Geometry check sheet. Reference: the model listing, model coordinates, mm. Round coordinates to 2 decimals unless told otherwise and drop trailing zeros. Loops run counter-clockwise (first coordinate to the right, second up) from the corner with the lowest first, then second, coordinate; pieces in that order, holes last. Notation, with made-up numbers: (-21, 20.5) -> (24, 20.5) arc R22 ccw to (24, 28.5) -> close; hole circle Ø7 at (17.5, -11). An arc over 180 degrees is marked (long way). Use a Markdown table: item, result. Add a question column.
Q1. Sectioned sample at D-D, the plane x = 1518.5. Enter the section's corners in (y, z).
Q2. Release check for a two-part mould opening along Z. For faces 1 (the face through (1175, -9, 335)), 2 (the face through (1360, -9, 10)), 3 (the face through (1361, -9, 344)), 4 (the face through (1360, -9, 670)) record: released by +Z, released by -Z, zero draft, split by the parting line, or undercut.
Q3. Material ranges on L1, parallel to X at y = -10, z = 461.5; L2, parallel to Y at x = 1386, z = 499.5; L3, parallel to Z at x = 1360, y = -13, recorded low to high.
Q4. Sectioned sample at A-A, the plane z = 313. Enter the section's corners in (x, y), then the cut area to 4 significant figures.
Q5. Sectioned sample at C-C, the plane z = 604.5. Enter the section's corners in (x, y), then the cut area to 4 significant figures.
Q6. Sectioned sample at B-B, the plane x = 1356. Enter the section's corners in (y, z), then the cut area to 3 significant figures.
```python
from build123d import *

# Parameters (mm, degrees)
CLONE2D002_W    = 375
CLONE2D002_H    = 660
PAD011_DEPTH    = 19
SKETCH027_W     = 225
SKETCH027_H     = 510
POCKET011_DEPTH = 10


with BuildPart() as part:
    # Clone2D002 → Pad011 (new body)
    with BuildSketch(Plane.XZ):
        with Locations((187.5, 330)):
            Rectangle(CLONE2D002_W, CLONE2D002_H)
    extrude(amount=PAD011_DEPTH)

    # Sketch027 (on Face6 of Pad011) → Pocket011 (cut)
    with BuildSketch(Plane.XZ.offset(19)):
        with Locations((187.5, 330)):
            Rectangle(SKETCH027_W, SKETCH027_H)
    extrude(amount=-POCKET011_DEPTH, mode=Mode.SUBTRACT)

    # Clone2D003 (on Face1 of Pocket011) → Revolution001 (revolve)
    with BuildSketch(Plane(origin=(40, -19, 330), x_dir=(-1, 0, 0), z_dir=(0, 0, -1))):
        with BuildLine():
            Line((0, 0), (0, -20))
            add(Edge.make_bspline(
                [(0, -20), (-18, -20), (-18, -9.133286), (-4.506424, -9.133286), (-7.5, 0)],
                knots=[0, 0, 0, 0, 0.5, 1, 1, 1, 1], degree=3, weights=[7, 6.116989, 5.810816, 6.060123, 5.999522]))
            Line((-7.5, 0), (0, 0))
        make_face()
    revolve(axis=Axis((40, -19, 330), (0, 1, 0)))


with BuildPart() as part_1:
    # Body011 placement: moved
    add(part.part.moved(Location((1175, 0, 10))))


solid = part_1.part
```
Values:
| question | item | result |
|---|---|---|
| 1 | outline | (-19, 10) -> (0, 10) -> (0, 670) -> (-19, 670) -> close |
| 2 | face 1 | zero draft |
| 2 | face 2 | released by -Z |
| 2 | face 3 | undercut |
| 2 | face 4 | released by +Z |
| 3 | L1 | 1175 to 1250, 1475 to 1550 |
| 3 | L2 | -9 to 0 |
| 3 | L3 | 10 to 85, 595 to 670 |
| 4 | outline | (1175, -19) -> (1250, -19) -> (1250, -9) -> (1475, -9) -> (1475, -19) -> (1550, -19) -> (1550, 0) -> (1175, 0) -> close |
| 4 | area | 4,875 mm^2 |
| 5 | outline | (1175, -19) -> (1550, -19) -> (1550, 0) -> (1175, 0) -> close |
| 5 | area | 7,125 mm^2 |
| 6 | outline | (-19, 10) -> (0, 10) -> (0, 670) -> (-19, 670) -> (-19, 595) -> (-9, 595) -> (-9, 85) -> (-19, 85) -> close |
| 6 | area | 7,440 mm^2 |
